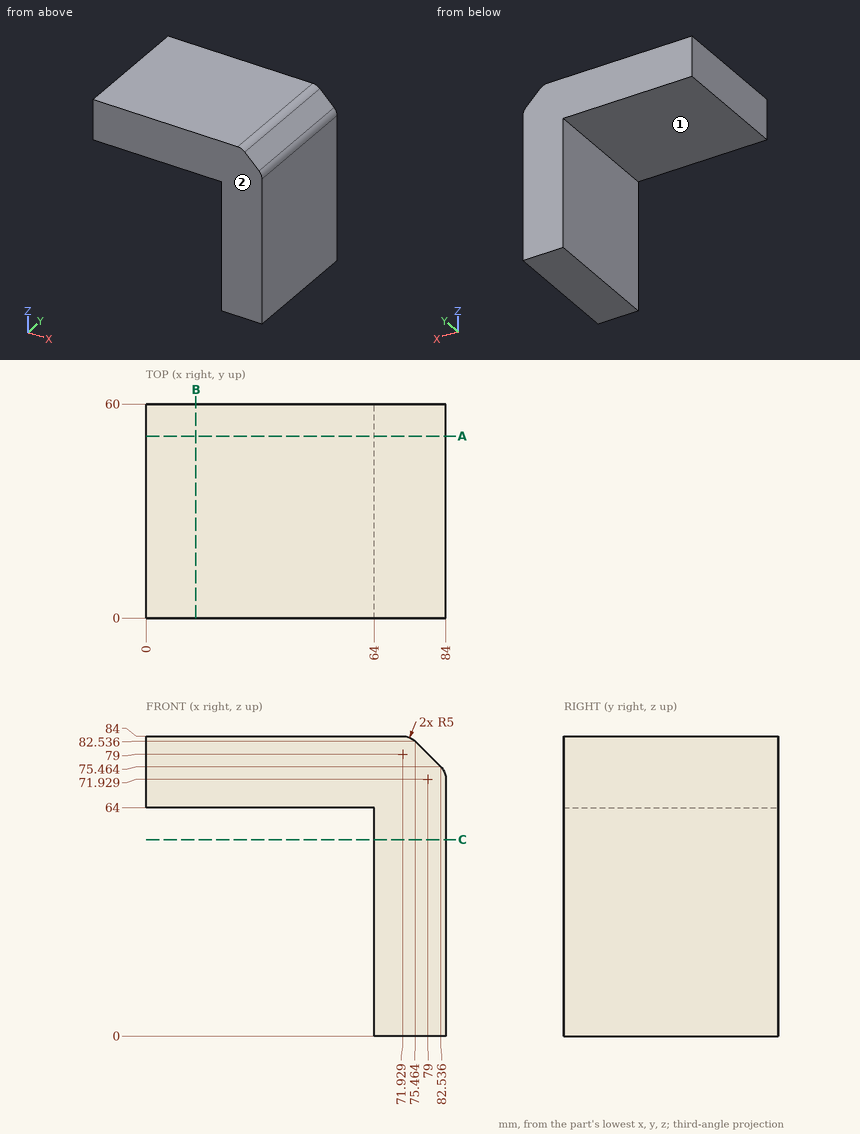
Study the drawing (mm; zero at the part's minimum x, y, z) and answer. A direction names the side the tool comes from. Round coordinates to 2 decimals unless told otherwise and drop trailing zeros. Order: outer loops, then holes, each group sorted by start corner. A loop starts at its lowest first (then second) coordinate and runs counter-clockwise, first axis right, second up. Notation, with made-up numbers: (28, 79.5) - (76, 79.5) arc R22 ccw to (76, 88.5) - close; hole circle Ø2 at (41, 30). An arc over 180 degrees is marked (long way). Use one line per item in the form item = value. Start each with the question number.
(1) For the marked faces 1 and 2, determine the directions among +Z, -Z, +X, -X, +Y, -Y from which every point of the face is accessible in a straight line to the end or side of a thin tool.
(2) The part is cut by section B-B (x = 14). Give the vertices of the cut face in (y, z), then the cut area to 3 significant figures.
(3) Find the intervals of material crossed by line 1 along X through (y, z) = (25, 43.5); line 2 along X through (y, z) = (39, 80.5), in increasing order. Write a range as from..to.
(4) Flat-ended cylindrical pins translate along their axes: pin 1 Ø3 at (x, y) = (74.5, 45) entering from +Z; pin 2 Ø12 at (x, y) = (29.5, 42.5) entering from -Z; pin 3 Ø10 at (y, z) = (28.5, 57) entering from -X. Find the tip coordinate at first contact, or state that the pin passes through.
(5) The part is cut by section A-A (y = 51). Give the vertices of the cut face in (x, z) (1 decimal).
(6) The part is cut by section C-C (z = 55). Give the vertices of the cut face in (x, y).
Checked values:
q1.face_1 = -Z, -X, +Y, -Y
q1.face_2 = +Z, -Z, +X, -X, -Y
q2.outline = (0, 64) - (60, 64) - (60, 84) - (0, 84) - close
q2.area = 1,200 mm^2
q3.line_1 = 64..84
q3.line_2 = 0..77.5
q4.pin_1 = 83.88
q4.pin_2 = 64
q4.pin_3 = 64
q5.outline = (0, 64) - (64, 64) - (64, 0) - (84, 0) - (84, 71.9) arc R5 ccw to (82.5, 75.5) - (75.5, 82.5) arc R5 ccw to (71.9, 84) - (0, 84) - close
q6.outline = (64, 0) - (84, 0) - (84, 60) - (64, 60) - close
